Build history of the part. All positions in model axes, mm. A direction names the side the tool comes from. Coordinates: 2 decimals unless noted, no trailing zeros. Loops run counter-clockwise (first coordinate to the right, second up) from the corner with the lowest first, then second, coordinate; pieces in that order, holes last. Notation, with made-up numbers: M -22,35.5 L 4,35.5 A21 cw 4,51.5 Z; hole C 41.25,52.5 d3. An arc over 180 degrees is marked long. Write each question's results on one line, items separated by ' | '. Start each with the question number.
Autodesk Inventor part; units mm, degrees
ref_plane "YZ Plane" through (0, 0, 0) normal (1, 0, 0) x (0, 1, 0)
ref_plane "XZ Plane" through (0, 0, 0) normal (0, 1, 0) x (-1, 0, 0)
ref_plane "XY Plane" through (0, 0, 0) normal (0, 0, 1) x (1, 0, 0)
sketch "Sketch1" plane through (0, 0, 0) normal (0, 1, 0) x (-1, 0, 0)
  line L0 (0, 20) -> (-92, 20)
  line L1 (-92, 20) -> (-92, -20)
  line L2 (-92, -20) -> (0, -20)
  line L3 (0, -20) -> (0, 20)
  line L4 (-46, 20) -> (-46, -20) construction
  line L5 (0, 0) -> (-92, 0) construction
  line L6 (0.15, 20.15) -> (-92.15, 20.15)
  line L7 (-92.15, 20.15) -> (-92.15, -20.15)
  line L8 (-92.15, -20.15) -> (0.15, -20.15)
  line L9 (0.15, -20.15) -> (0.15, 20.15)
  dimension "d0" = 40
  dimension "d1" = 92
  dimension "d19" = 0.15
extrude "Extrusion1" add sketch "Sketch1" along normal blind 0.7 contours L3 L2 L1 L0 | L9 L8 L7 L6
sketch "Sketch2" plane through (0, 0.7, 0) normal (0, 1, 0) x (1, 0, 0)
  line L0 (92.15, -20.15) -> (92.15, 20.15)
  line L1 (92.15, 20.15) -> (-0.15, 20.15)
  line L2 (-0.15, 20.15) -> (-0.15, -20.15)
  line L3 (-0.15, -20.15) -> (92.15, -20.15)
  line L4 (1.05, -18.95) -> (1.05, 18.95)
  line L5 (1.05, 18.95) -> (90.95, 18.95)
  line L6 (90.95, 18.95) -> (90.95, -18.95)
  line L7 (90.95, -18.95) -> (1.05, -18.95)
  dimension "d20" = 1.2
extrude "Extrusion2" add sketch "Sketch2" along normal blind 5.5
sketch "Sketch4" plane through (0, 0, 0) normal (0, 1, 0) x (1, 0, 0)
  line L0 (1.05, -18.95) -> (90.95, -18.95)
  line L1 (90.95, -18.95) -> (90.95, 18.95)
  line L2 (90.95, 18.95) -> (1.05, 18.95)
  line L3 (1.05, 18.95) -> (1.05, -18.95)
  line L4 (92.15, 20.15) -> (-0.15, 20.15)
  line L5 (-0.15, 20.15) -> (-0.15, -20.15)
  line L6 (-0.15, -20.15) -> (92.15, -20.15)
  line L7 (92.15, -20.15) -> (92.15, 20.15)
  line L8 (1.05, -18.95) -> (1.05, 18.95)
  line L9 (1.05, 18.95) -> (90.95, 18.95)
  line L10 (90.95, 18.95) -> (90.95, -18.95)
  line L11 (90.95, -18.95) -> (1.05, -18.95)
  circle A0 centre (2.55, -17.45) radius 1.5
  circle A1 centre (2.55, 17.45) radius 1.5
  circle A2 centre (89.45, 17.45) radius 1.5
  line L12 (-1.15, -21.15) -> (-1.15, 21.15)
  line L13 (-1.15, 21.15) -> (93.15, 21.15)
  line L14 (93.15, 21.15) -> (93.15, -21.15)
  line L15 (93.15, -21.15) -> (-1.15, -21.15)
  line L16 (-0.15, 20.15) -> (-1.15, 20.15)
  line L17 (-0.15, -20.15) -> (-1.15, -20.15)
  line L18 (2.55, -17.45) -> (1.05, -17.45)
  line L19 (2.55, -17.45) -> (2.55, -18.95)
  line L20 (2.55, 17.45) -> (2.55, 18.95)
  line L21 (2.55, 17.45) -> (1.05, 17.45)
  line L22 (89.45, 17.45) -> (89.45, 18.95)
  line L23 (89.45, 17.45) -> (90.95, 17.45)
  circle A3 centre (2.55, -17.55) radius 1.6
  point P0 (0, 0)
  dimension "d21" = 3
  dimension "d22" = 3
  dimension "d24" = 3
  dimension "d25" = 2.7
  dimension "d26" = 2.7
  dimension "d28" = 2.7
  dimension "d29" = 1
extrude "Extrusion3" add sketch "Sketch4" along normal blind 8 contours L19 L18 A0 | A0 L18 L19 | L21 L20 A1 | A1 L20 L21 | L23 L22 A2 | A2 L22 L23 | L4 L16 L12 L13 L14 L15 L17 L6 L7 | L5 L17 L12 L16
sketch "Sketch7" plane through (0, 8, 0) normal (0, 1, 0) x (1, 0, 0)
  line L0 (0.05, 14.425) -> (6.05, 14.425)
  line L1 (0.05, 0.525) -> (6.05, 0.525)
  line L2 (-1.15, 21.15) -> (-1.15, -21.15)
  line L3 (-1.15, -21.15) -> (93.15, -21.15)
  line L4 (93.15, -21.15) -> (93.15, 21.15)
  line L5 (93.15, 21.15) -> (-1.15, 21.15)
  line L6 (-0.15, 20.15) -> (92.15, 20.15)
  line L7 (92.15, 20.15) -> (92.15, -20.15)
  line L8 (92.15, -20.15) -> (-0.15, -20.15)
  line L9 (-0.15, -20.15) -> (-0.15, 20.15)
  line L10 (-0.15, 20.15) -> (-0.15, -20.15)
  line L11 (-1.15, 21.15) -> (-1.15, -21.15)
  line L12 (-0.15, 15.425) -> (-1.15, 15.425)
  line L13 (-1.15, 15.425) -> (-1.15, -0.475)
  line L14 (-1.15, -0.475) -> (-0.15, -0.475)
  line L15 (-0.15, -0.475) -> (-0.15, 15.425)
  point P0 (0, 0)
  point P1 (-0.15, -0.475)
  point P2 (-1.15, 15.425)
  dimension "d32" = 1
  dimension "d33" = 1
extrude "Extrusion4" cut sketch "Sketch7" against normal blind 0.4 contours L12 L9 L14 L2
sketch "Sketch8" plane through (0, 0.7, 0) normal (0, 1, 0) x (1, 0, 0)
  circle A0 centre (55.0598, -12.05) radius 4.4577
  circle A1 centre (60.1398, -17.13) radius 0.9906
  circle A2 centre (49.9798, -6.97) radius 0.9906
  circle A3 centre (49.9798, -6.97) radius 0.8406
  circle A4 centre (60.1398, -17.13) radius 0.8406
  point P0 (0, 0)
  dimension "d37" = 0.15
  dimension "d38" = 0.15
extrude "Extrusion5" [suppressed]
sketch "Sketch9" plane through (0, 0.7, 0) normal (0, 1, 0) x (1, 0, 0)
  arc A0 (1.05, 17.45) -> (2.55, 18.95) centre (2.55, 17.45) ccw
  arc A1 (89.45, 18.95) -> (90.95, 17.45) centre (89.45, 17.45) ccw
  arc A2 (1.05, -17.45) -> (2.55, -18.95) centre (2.55, -17.45) ccw
  line L0 (90.95, 18.95) -> (89.45, 18.95)
  line L1 (1.05, 18.95) -> (1.05, 17.45)
  circle A3 centre (2.55, 17.45) radius 1.5
  circle A4 centre (2.55, -17.45) radius 1.5
  circle A5 centre (89.45, -17.45) radius 1.5
  circle A6 centre (89.45, 17.45) radius 1.5
  line L2 (2.55, 17.45) -> (1.05, 17.45)
  line L3 (2.55, 17.45) -> (2.55, 18.95)
  line L4 (89.45, 17.45) -> (89.45, 18.95)
  line L5 (89.45, 17.45) -> (90.95, 17.45)
  line L6 (89.45, -17.45) -> (89.45, -18.95)
  line L7 (89.45, -17.45) -> (90.95, -17.45)
  line L8 (2.55, -17.45) -> (1.05, -17.45)
  line L9 (2.55, -17.45) -> (2.55, -18.95)
  line L10 (1.05, 17.45) -> (1.05, -17.45)
  arc A7 (2.55, -18.95) -> (1.05, -17.45) centre (2.55, -17.45) ccw
  line L11 (2.55, -18.95) -> (90.95, -18.95)
  line L12 (90.95, -18.95) -> (90.95, 17.45)
  line L13 (89.45, 18.95) -> (2.55, 18.95)
  arc A8 (2.55, 18.95) -> (1.05, 17.45) centre (2.55, 17.45) ccw
  line L14 (2.55, 18.95) -> (1.05, 18.95)
  arc A9 (90.95, 17.45) -> (89.45, 18.95) centre (89.45, 17.45) ccw
  line L15 (90.95, 17.45) -> (90.95, 18.95)
  line L16 (1.05, -17.45) -> (1.05, -18.95)
  line L17 (1.05, -18.95) -> (2.55, -18.95)
  point P0 (0, 0)
  point P1 (90.95, 17.45)
  point P2 (89.45, 18.95)
  point P3 (2.55, 18.95)
  point P4 (1.05, 17.45)
  point P5 (2.55, -18.95)
  point P6 (1.05, -17.45)
extrude "Extrusion6" add sketch "Sketch9" along normal up to surface (5.5 mm away) contours L1 L14 A3 | A0 L13 A1 L12 A5 L11 A4 L10 | L8 L9 A2 | A4 L9 L8 | A2 L17 L16 | L0 L15 A6 | L6 L7 A5 | A5 L7 L6 | A5 L12 L11
fillet "Fillet1" radius 1 4 edges at (-1.15, 4, 21.15) (93.15, 4, 21.15) (93.15, 4, -21.15) (-1.15, 4, -21.15)
equation "\"d22\" = d21"
equation "\"d24\" = d21"
equation "\"d26\" = d25"
equation "\"d28\" = d25"
equation "\"d33\" = d32"
properties part number "base"
1. Mould opens along Z. For faces 1 (the flat face through (45, 7, 20.15)), 2 (the flat face through (3, 8, -17)), 3 (the flat face through (47, 4, 21.15)), 4 (the flat face through (92.15, 7, 0)) say: +Z half, -Z half, draft (parallel to the pull), parting line (faces both ways), or undercut.
2. Band-saw the part on D-D, the plane x = 89.45. List the corners of the cut face in (y, z), plus the area to 3 significant figures.
3. Band-saw the part on A-A, the plane x = 70. List the corners of the cut face in (y, z).
4. Band-saw the part on B-B, the plane z = -17.45. List the corners of the cut face in (x, y).
5. Which spindle directions (+Z, -Z, +X, -X, +Y, -Y) get a long thin tool onto all of the face, cutting with end or side? Do faces 5 (the flat face through (45.8, 8, -20.5)), 6 (the cylindrical face through (1.44, 7.09, 18.46)). Say none if no direction does.
6. Band-saw the part on C-C, the plane z = 17.45. List the corners of the cut face in (x, y), plus the area to 3 significant figures.
7. Wall check: line 1 along Z through (x, y) = (40, 6.5); line 2 along Y through (x, z) = (44.5, -12). Give the ranges that are in metal, low to high.
8. Pin check, flat tips, straight feed: pin 1 (0.5 mm diameter, centred on x = -0.5, z = -8.5, fed in from +Y); pin 2 (2 mm diameter, centred on x = 41.5, z = -5.5, fed in from +Y). Stop position of each tip, or through.
Checked values:
1) face 1: undercut | face 2: draft | face 3: +Z half | face 4: undercut
2) outline: M 0,-21.15 L 8,-21.15 L 8,-20.15 L 6.2,-20.15 L 6.2,-18.95 L 8,-18.95 L 8,-15.95 L 6.2,-15.95 L 6.2,20.15 L 8,20.15 L 8,21.15 L 0,21.15 Z | area: 271 mm²
3) outline: M 0,-21.15 L 8,-21.15 L 8,-20.15 L 6.2,-20.15 L 6.2,20.15 L 8,20.15 L 8,21.15 L 0,21.15 Z
4) outline: M -1.15,0 L 93.15,0 L 93.15,8 L 92.15,8 L 92.15,6.2 L 90.95,6.2 L 90.95,8 L 87.95,8 L 87.95,6.2 L 4.05,6.2 L 4.05,8 L 1.05,8 L 1.05,6.2 L -0.15,6.2 L -0.15,8 L -1.15,8 Z
5) face 5: +Z, -Z, +X, -X, +Y | face 6: +Y
6) outline: M -1.15,0 L 93.15,0 L 93.15,8 L 92.15,8 L 92.15,6.2 L 4.05,6.2 L 4.05,8 L 1.05,8 L 1.05,6.2 L -0.15,6.2 L -0.15,8 L -1.15,8 Z | area: 594 mm²
7) line 1: -21.15 to -20.15, 20.15 to 21.15 | line 2: 0 to 6.2
8) pin 1: y = 7.6 | pin 2: y = 6.2
